For this review, use the dimensioned drawing (mm, ordinates from the lowest corner) and the shaded views. A direction names the side the tool comes from. Coordinates: 2 decimals unless noted, no trailing zeros. Loops run counter-clockwise (first coordinate to the right, second up) from the corner with the lowest first, then second, coordinate; pieces in that order, holes last. Notation, with made-up numbers: (19, -9.75) - (78, -9.75) arc R10 ccw to (78, 8.25) - close; hole circle Ø10 at (-22, 84). An arc over 180 degrees is marked (long way). One line per item, written item: value. Start each with the question number.
1. Insertion check: P1, Ø12, axis at y = 12.5, z = 36.5, coming from the +X side; P2, Ø2, axis at y = 19, z = 34, coming from the -X side; P3, Ø10, axis at x = 18.5, z = 8, coming from the -Y side; P4, Ø8, axis at x = 29.5, y = 26.5, coming from the +Z side. Each pin has a flat end and moves straight along its axis. Give the tip position at first contact, or say it passes through.
2. We need section A-A, the plane x = 12.5. Give the boundary of the cut face in (y, z).
3. We need section C-C, the plane x = 16. Give the boundary of the cut face in (y, z).
4. We need section D-D, the plane z = 8.5. Give the boundary of the cut face in (x, y), then the cut area to 3 significant figures.
5. Mouldability with a two-part tool opening along Z and no side actions: class the marked faces 1, 2, 3 and 4 as +Z half, -Z half, draft (parallel to the pull), parting line (faces both ways), or undercut.
6. To check wall thickness, follow line 1 (Z direction, x = 3, y = 26.5); line 2 (Z direction, x = 31, y = 2); line 3 (X direction, y = 25.25, z = 29.5). State the ranges of each line that lie inside material, in increasing order.
7. For the marked faces 5 and 6, list the 3-axis set-ups (+Z, -Z, +X, -X, +Y, -Y) from which the entire face can be reached by the end or side of a thin tool; tool diameter is ignored.
8. We need section B-B, the plane y = 26. Give the boundary of the cut face in (x, z), then the cut area to 3 significant figures.
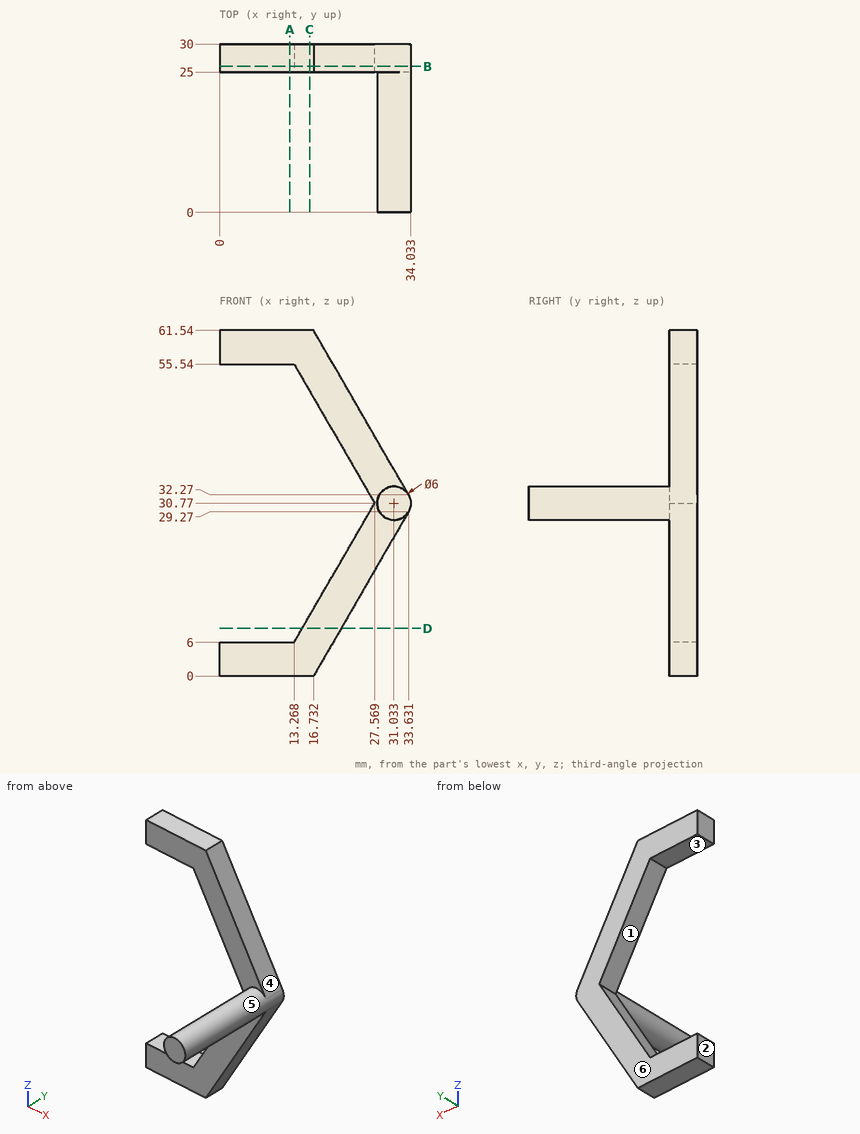
Findings below:
1. P1: x = 34.03
1. P2: x = 29.03
1. P3: y = 25
1. P4: z = 46.35
2. outline: (25, 0) - (30, 0) - (30, 6) - (25, 6) - close; (25, 55.54) - (30, 55.54) - (30, 61.54) - (25, 61.54) - close
3. outline: (25, 0) - (30, 0) - (30, 10.73) - (25, 10.73) - close; (25, 50.81) - (30, 50.81) - (30, 61.54) - (25, 61.54) - close
4. outline: (14.71, 25) - (21.64, 25) - (21.64, 30) - (14.71, 30) - close
4. area: 34.6 mm2
5. face 1: undercut
5. face 2: draft
5. face 3: undercut
5. face 4: +Z half
6. line 1: 0 to 6, 55.54 to 61.54
6. line 2: 27.77 to 33.77
6. line 3: 26.84 to 33.75
7. face 5: -Y
7. face 6: +Z, -Z, +X, -X, +Y
8. outline: (0, 0) - (16.73, 0) - (33.63, 29.27) arc R3 ccw to (33.63, 32.27) - (16.73, 61.54) - (0, 61.54) - (0, 55.54) - (13.27, 55.54) - (27.57, 30.77) - (13.27, 6) - (0, 6) - close
8. area: 564 mm2
